Part print with two shaded views. Sizes in mm from the minimum x, y, z corner. A direction names the side the tool comes from. Give positions to 0.01 mm unless a question says otherwise; leave off trailing zeros. Write each loop counter-clockwise with the first axis right and the second up, starting at its lowest first coordinate (ties: lowest second). Pieces come first, ordered by that corner, then holes.
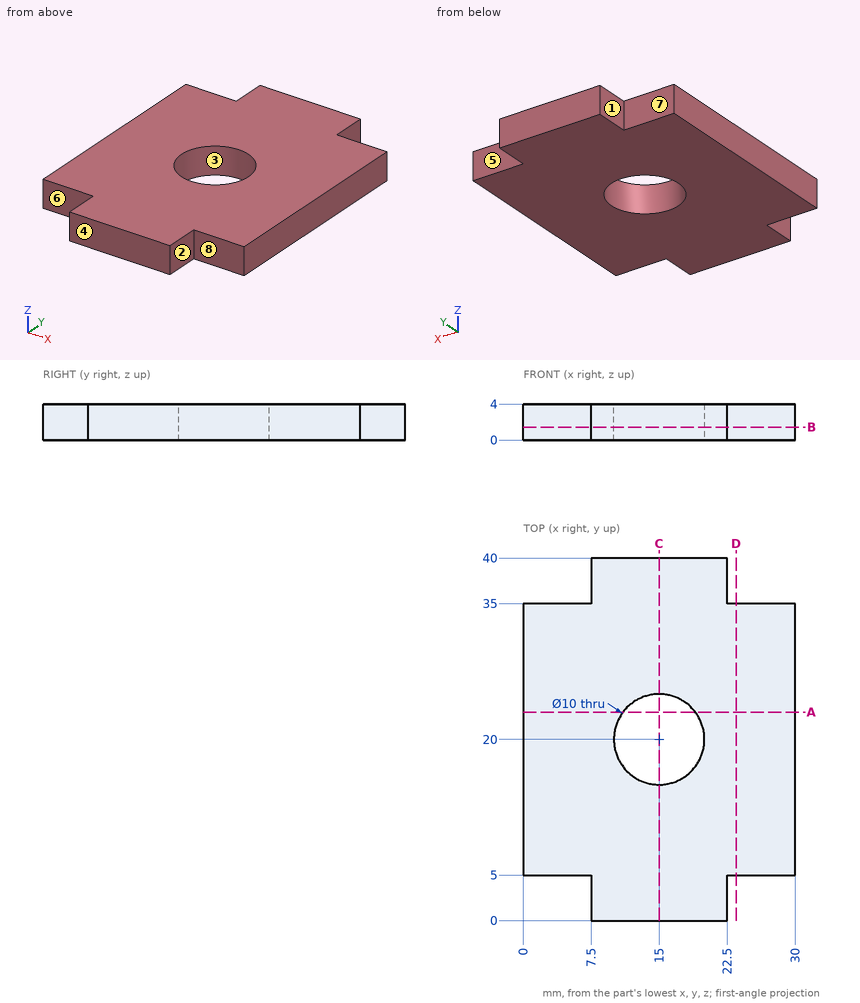
1) Saw through at D-D (x = 23.5). Write the cut outline in (y, z).
Check result:
outline: (5, 0) - (35, 0) - (35, 4) - (5, 4) - close
2) Drill centre lines: L1, parallel to Y at x = 15, z = 1.1; L2, parallel to Y at x = 28.5, z = 1.5; L3, parallel to X at y = 15.5, z = 2.7. Where is each one in solid material? Low to high.
Check result:
L1: y = 0 to 15, 25 to 40
L2: y = 5 to 35
L3: x = 0 to 12.82, 17.18 to 30
3) Saw through at C-C (x = 15). Write the cut outline in (y, z), and give its area (3 significant figures).
Check result:
outline: (0, 0) - (15, 0) - (15, 4) - (0, 4) - close; (25, 0) - (40, 0) - (40, 4) - (25, 4) - close
area: 120 mm2
4) Mould opens along X. For the marked faces 1, 2, 3 and 4 say: +X half, -X half, draft (parallel to the pull), parting line (faces both ways), or undercut.
Check result:
face 1: -X half
face 2: +X half
face 3: undercut
face 4: draft
5) Saw through at B-B (z = 1.45). Write the cut outline in (x, y), and give its area (3 significant figures).
Check result:
outline: (0, 5) - (7.5, 5) - (7.5, 0) - (22.5, 0) - (22.5, 5) - (30, 5) - (30, 35) - (22.5, 35) - (22.5, 40) - (7.5, 40) - (7.5, 35) - (0, 35) - close; hole circle Ø10 at (15, 20)
area: 971 mm2
6) Flat gauge pin, fed straight in: P1, Ø1.2, axis at y = 36.5, z = 1, coming from the -X side. Where does the tip first touch, or does it go through?
Check result:
P1: stops at x = 7.5
7) Saw through at A-A (y = 23). Write the cut outline in (x, z), and give its area (3 significant figures).
Check result:
outline: (0, 0) - (11, 0) - (11, 4) - (0, 4) - close; (19, 0) - (30, 0) - (30, 4) - (19, 4) - close
area: 88.0 mm2
8) 3-axis set-ups, long thin cutter, end or side, ignore diameter. For the marked faces 5, 6, 7 and 8: which of +Z, -Z, +X, -X, +Y, -Y reach the whole face in a straight line?
Check result:
face 5: +Z, -Z, +X, +Y
face 6: +Z, -Z, -X, -Y
face 7: +Z, -Z, -X, +Y
face 8: +Z, -Z, +X, -Y
